Verification items for the finished model (mm, model axes). A direction names the side the tool comes from. Give positions to 0.01 mm unless a question says otherwise; leave off trailing zeros. Loops run counter-clockwise (first coordinate to the right, second up) from the corner with the lowest first, then second, coordinate; pieces in that order, holes last. Notation, with made-up numbers: (-17, 28.25) - (-13, 28.25) arc R11 cw to (-13, 33.25) - close; hole circle Ø7 at (-26, 26.25). An arc over 180 degrees is marked (long way). Answer in a Markdown table with one row per item.
```python
from build123d import *


with BuildPart() as part:
    # Sweep1: sweep along a path in Sketch2
    with BuildLine(Plane.XY) as sweep1_path:
        Line((304.8, 609.6), (-304.8, 609.6))
        Line((-304.8, 609.6), (-304.8, 0))
        Line((-304.8, 0), (304.8, 0))
        Line((304.8, 0), (304.8, 609.6))
    # Sketch1 → Sweep1 (sweep)
    with BuildSketch(Plane(origin=(0, 0, 0), x_dir=(0, 0, -1), z_dir=(1, 0, 0))):
        Polygon((-12.7, -6.35), (-17.4625, -6.35), (-17.4625, 6.35), (4.7625, 6.35), (4.7625, 11.1125), (11.1125, 11.1125), (11.1125, 9.525), (17.4625, 9.525), (17.4625, -6.35), (12.7, -6.35), (12.7, 0), (-12.7, 0), align=None)
    sweep(path=sweep1_path.line, transition=Transition.RIGHT)


solid = part.part
```
Q1. Thickness scan on line 1 (Y direction, x = -269, z = 3.5); line 2 (X direction, y = 254, z = 15); line 3 (Y direction, x = -79.5, z = 16). Record the ranges inside material, lowest first.
Completed:
| item | result |
|---|---|
| line 1 | 0 to 6.35, 603.25 to 609.6 |
| line 2 | -311.15 to -298.45, 298.45 to 311.15 |
| line 3 | -6.35 to 6.35, 603.25 to 615.95 |
Q2. Tool access check on faces 1 (the face through (-298.45, 301, 6)), 2 (the face through (-304.8, 301, 0)), 3 (the face through (304.8, 309, 0)), 4 (the face through (-4, 609.6, 0)), 5 (the face through (-140, 4, 17.463)). Record the directions out of +Z, -Z, +X, -X, +Y, -Y that give a thin tool (end or side, any length) a straight path to the whole face; none if there is none.
Completed:
| item | result |
|---|---|
| face 1 | +Z |
| face 2 | -X, +Y, -Y |
| face 3 | +X, +Y, -Y |
| face 4 | +X, -X, +Y |
| face 5 | +Z, +X, -X, +Y, -Y |
Q3. Go/stop test with flat-tipped pins: P1, Ø5, axis at y = 436.5, z = -6.5, coming from the +X side; P2, Ø2, axis at y = 503.5, z = -11, coming from the -X side; P3, Ø12.5, axis at x = -4.5, z = -0.5, coming from the +Y side. Record where each tip stops, or that it passes through.
Completed:
| item | result |
|---|---|
| P1 | x = 304.8 |
| P2 | x = -304.8 |
| P3 | y = 609.6 |
Q4. Sectioned sample at B-B (z = 5.5). Record the cut outline in (x, y), and give its area (3 significant figures).
Completed:
| item | result |
|---|---|
| outline | (-304.8, 0) - (304.8, 0) - (304.8, 609.6) - (-304.8, 609.6) - close; hole (-298.45, 6.35) - (298.45, 6.35) - (298.45, 603.25) - (-298.45, 603.25) - close |
| area | 15,300 mm^2 |
Q5. Draft check along Z on faces 6 (the face through (4, 0, 0)), 7 (the face through (298, 329, -17.462)), 8 (the face through (4, 6.35, 6)). Enter one of: +Z half, -Z half, draft (parallel to the pull), parting line (faces both ways), or undercut.
Completed:
| item | result |
|---|---|
| face 6 | undercut |
| face 7 | -Z half |
| face 8 | draft |
